Read the model definition and answer for the solid it produces. Units are mm, in the model's axes. A direction names the side the tool comes from. Give positions to 0.01 mm unless a question says otherwise; leave off trailing zeros. Order: outer loops, then holes, each group sorted by start corner. A loop starts at its lowest first (then second) coordinate and runs counter-clockwise, first axis right, second up. Notation, with made-up numbers: (23.25, 27.5) -> (72.25, 27.5) arc R16 cw to (72.25, 50.5) -> close; hole circle Ø5 at (-26, 3). An arc over 180 degrees is marked (long way). One line per item, written item: value. Start each with the question number.
from build123d import *

# Parameters (mm, degrees)
SKETCH1_R           = 1.6
SKETCH1_R_2         = 20
SKETCH1_R_3         = 3
BOSS_EXTRUDE1_DEPTH = 5
FILLET1_R           = 5
SKETCH4_R           = 3.25
CUT_EXTRUDE2_DEPTH  = 1.5


with BuildPart() as part:
    # Sketch1 → Boss-Extrude1 (new body)
    with BuildSketch(Plane(origin=(0, 0, 0), x_dir=(1, 0, 0), z_dir=(0, 1, 0))):
        with BuildLine():
            Line((-75, 35), (0, 35))
            ThreePointArc((0, 35), (35, 0), (0, -35))
            Line((0, -35), (-75, -35))
            Line((-75, -35), (-75, 35))
        make_face()
        with Locations((0, 25)):
            Circle(SKETCH1_R, mode=Mode.SUBTRACT)
        with Locations((21.650635095, 12.5)):
            Circle(SKETCH1_R, mode=Mode.SUBTRACT)
        with Locations((21.650635095, -12.5)):
            Circle(SKETCH1_R, mode=Mode.SUBTRACT)
        with Locations((0, -25)):
            Circle(SKETCH1_R, mode=Mode.SUBTRACT)
        with Locations((-21.650635095, -12.5)):
            Circle(SKETCH1_R, mode=Mode.SUBTRACT)
        with Locations((-21.650635095, 12.5)):
            Circle(SKETCH1_R, mode=Mode.SUBTRACT)
        Circle(SKETCH1_R_2, mode=Mode.SUBTRACT)
        with Locations((-67.5, 5)):
            Circle(SKETCH1_R, mode=Mode.SUBTRACT)
        with Locations((-52.5, 5)):
            Circle(SKETCH1_R, mode=Mode.SUBTRACT)
        with Locations((-52.5, -5)):
            Circle(SKETCH1_R, mode=Mode.SUBTRACT)
        with Locations((-67.5, -5)):
            Circle(SKETCH1_R, mode=Mode.SUBTRACT)
        with Locations((-60, 20)):
            Circle(SKETCH1_R_3, mode=Mode.SUBTRACT)
        with Locations((-60, -20)):
            Circle(SKETCH1_R_3, mode=Mode.SUBTRACT)
    extrude(amount=BOSS_EXTRUDE1_DEPTH)

    # Fillet1
    fillet1_edges = [part.edges().sort_by_distance(p)[0] for p in [
        (-75, 2.5, -35),
        (-75, 2.5, 35),
    ]]
    fillet(fillet1_edges, radius=FILLET1_R)

    # Sketch4 → Cut-Extrude2 (cut)
    with BuildSketch(Plane.XZ):
        with Locations((0, 25)):
            Circle(SKETCH4_R)
        with Locations((21.650635095, 12.5)):
            Circle(SKETCH4_R)
        with Locations((21.650635095, -12.5)):
            Circle(SKETCH4_R)
        with Locations((0, -25)):
            Circle(SKETCH4_R)
        with Locations((-21.650635095, -12.5)):
            Circle(SKETCH4_R)
        with Locations((-21.650635095, 12.5)):
            Circle(SKETCH4_R)
    extrude(amount=-CUT_EXTRUDE2_DEPTH, mode=Mode.SUBTRACT)


solid = part.part
Item 1: Find section A-A on x = -60. Write down the section's boundary in (y, z).
Item 2: Find the intervals of material crossed by line 1 (Z direction, x = -60, y = 2); line 2 (Z direction, x = -67.5, y = 2.15); line 3 (X direction, y = 3.15, z = 0), in increasing order. Write a range as from..to.
Item 3: A tool of negligible diameter and unlimited length cuts with its end or side. For faces 1 (the cylindrical face through (-50.974, 2.465, 4.519)), 2 (the flat face through (23, 1.5, 11)), from which of +Z, -Z, +X, -X, +Y, -Y can it reach the whole face along a straight path? Write none if from no direction.
Item 4: Find section B-B on z = 0. Write down the section's boundary in (x, y), then the cut area to 3 significant figures.
Item 5: Find section D-D on z = 12.5. Write down the section's boundary in (x, y), then the cut area to 3 significant figures.
Item 6: Find section C-C on x = -7. Write down the section's boundary in (y, z) (3 decimals), then the cut area to 3 significant figures.
Item 7: Flat-ended cylindrical pins translate along their axes: pin 1 (2 mm diameter, centred on x = 17, y = 3.5, fed in from -Z); pin 2 (2.5 mm diameter, centred on x = -52.5, z = -5, fed in from -Y); pin 3 (2 mm diameter, centred on x = 21, z = 11.5, fed in from -Y). Find the tip coordinate at first contact, or state that the pin passes through.
Item 8: For a pull along X with two mould halves and no side action, classify faces 3 (the cylindrical face through (24.75, 0.74, -11.52)), 4 (the flat face through (23, 1.5, -14)), 5 (the flat face through (-31, 0, 0)), 6 (the flat face through (-75, 2, 0)) as +X half, -X half, draft (parallel to the pull), parting line (faces both ways), or undercut.
Checks:
1. outline: (0, -35) -> (5, -35) -> (5, -23) -> (0, -23) -> close; (0, -17) -> (5, -17) -> (5, 17) -> (0, 17) -> close; (0, 23) -> (5, 23) -> (5, 35) -> (0, 35) -> close
2. line 1: -35..-23, -17..17, 23..35
2. line 2: -35..-6.6, -3.4..3.4, 6.6..35
2. line 3: -75..-20, 20..35
3. face 1: +Y, -Y
3. face 2: -Y
4. outline: (-75, 0) -> (-20, 0) -> (-20, 5) -> (-75, 5) -> close; (20, 0) -> (35, 0) -> (35, 5) -> (20, 5) -> close
4. area: 350 mm2
5. outline: (-75, 0) -> (-24.9, 0) -> (-24.9, 1.5) -> (-23.25, 1.5) -> (-23.25, 5) -> (-75, 5) -> close; (-20.05, 1.5) -> (-18.4, 1.5) -> (-18.4, 0) -> (-15.61, 0) -> (-15.61, 5) -> (-20.05, 5) -> close; (15.61, 0) -> (18.4, 0) -> (18.4, 1.5) -> (20.05, 1.5) -> (20.05, 5) -> (15.61, 5) -> close; (23.25, 1.5) -> (24.9, 1.5) -> (24.9, 0) -> (32.69, 0) -> (32.69, 5) -> (23.25, 5) -> close
5. area: 340 mm2
6. outline: (0, -35) -> (5, -35) -> (5, -18.735) -> (0, -18.735) -> close; (0, 18.735) -> (5, 18.735) -> (5, 35) -> (0, 35) -> close
6. area: 163 mm2
7. pin 1: z = -31.13
7. pin 2: through
7. pin 3: y = 1.5
8. face 3: undercut
8. face 4: undercut
8. face 5: draft
8. face 6: -X half
